Autodesk Inventor part; units mm, degrees
ref_plane "YZ Plane" through (0, 0, 0) normal (1, 0, 0) x (0, 1, 0)
ref_plane "XZ Plane" through (0, 0, 0) normal (0, 1, 0) x (-1, 0, 0)
ref_plane "XY Plane" through (0, 0, 0) normal (0, 0, 1) x (1, 0, 0)
sketch "Sketch1" plane through (0, 0, 0) normal (0, 0, 1) x (1, 0, 0)
  line L0 (-19.05, -19.05) -> (19.05, -19.05)
  line L1 (19.05, -19.05) -> (19.05, 19.05)
  line L2 (19.05, 19.05) -> (-19.05, 19.05)
  line L3 (-19.05, 19.05) -> (-19.05, -19.05)
  line L4 (-19.05, -19.05) -> (19.05, 19.05) construction
  line L5 (19.05, -19.05) -> (-19.05, 19.05) construction
  line L6 (-15.875, -15.875) -> (15.875, -15.875)
  line L7 (15.875, -15.875) -> (15.875, 15.875)
  line L8 (15.875, 15.875) -> (-15.875, 15.875)
  line L9 (-15.875, 15.875) -> (-15.875, -15.875)
  line L10 (-15.875, -15.875) -> (15.875, 15.875) construction
  line L11 (15.875, -15.875) -> (-15.875, 15.875) construction
  point P0 (0, 0)
  dimension "d0" = 38.1
  dimension "d1" = 3.175
extrude "Extrusion1" add sketch "Sketch1" along normal mid plane 304.8
sketch "Sketch3" plane through (0, 0, 152.4) normal (0, 0, 1) x (1, 0, 0)
  line L0 (-19.05, -19.05) -> (19.05, -19.05)
  line L1 (19.05, -19.05) -> (19.05, 19.05)
  line L2 (19.05, 19.05) -> (-19.05, 19.05)
  line L3 (-19.05, 19.05) -> (-19.05, -19.05)
  line L4 (-19.05, -19.05) -> (19.05, 19.05) construction
  line L5 (19.05, -19.05) -> (-19.05, 19.05) construction
  point P0 (0, 0)
extrude "Extrusion2" add sketch "Sketch3" along normal blind 3.175
sketch "Sketch4" plane through (0, 0, 155.575) normal (0, 0, 1) x (1, 0, 0)
  point P0 (0, 0)
  point P1 (0, 0)
hole "Hole1" at (0, 0, 155.575) direction (0, 0, -1) diameter 6.35 end through all
properties part number "LinearExample"
Could you check a few things on this model? Use its own coordinates, in mm. A direction names the side the tool comes from. Give positions to 0.01 mm unless a question says otherwise; leave off trailing zeros. Order: outer loops, then holes, each group sorted by start corner. A loop starts at its lowest first (then second) coordinate and runs counter-clockwise, first axis right, second up.
Item 1: If we mould it in two halves opening along Y, with no side actions, what happens to faces 1 (the face through (-17, 0, -152.4)), 2 (the face through (3.1, 0.69, 153.97)), 3 (the face through (0, -19.05, -1))? For each: pulls with the +Y half, pulls with the -Y half, needs draft (parallel to the pull), parting line crosses it, or undercut.
Item 2: If we section it at C-C, the plane z = -91: Write out the boundary of the cut face in (x, y) (3 decimals).
Item 3: I'm going to push a flat-ended pin straight in: pin 1 (9.5 mm diameter, centred on x = -5.5, y = -7, fed in from -Z). Where does the tip first touch, or does it pass through?
Item 4: If we section it at A-A, the plane x = 0: Write out the boundary of the cut face in (y, z) (3 decimals), plus the area to 3 significant figures.
Item 5: I need wall thicknesses on line 1 (X direction, y = 0, z = 154.1) (3 decimals); line 2 (X direction, y = 9, z = -87) (3 decimals). Which ranges of each line are inside material? Lowest first, please.
Item 6: For faces 4 (the face through (19.05, 0, -1)), 5 (the face through (0, 15.875, -2)), which set-ups out of +Z, -Z, +X, -X, +Y, -Y let a thin tool reach every point of the face, with its end or its side?
Values:
1. face 1: needs draft
1. face 2: undercut
1. face 3: pulls with the -Y half
2. outline: (-19.05, -19.05) - (19.05, -19.05) - (19.05, 19.05) - (-19.05, 19.05) - close; hole (-15.875, -15.875) - (15.875, -15.875) - (15.875, 15.875) - (-15.875, 15.875) - close
3. pin 1: stops at z = 152.4
4. outline: (-19.05, -152.4) - (-15.875, -152.4) - (-15.875, 152.4) - (-3.175, 152.4) - (-3.175, 155.575) - (-19.05, 155.575) - close; (3.175, 152.4) - (15.875, 152.4) - (15.875, -152.4) - (19.05, -152.4) - (19.05, 155.575) - (3.175, 155.575) - close
4. area: 2,040 mm2
5. line 1: x = -19.05 to -3.175, 3.175 to 19.05
5. line 2: x = -19.05 to -15.875, 15.875 to 19.05
6. face 4: +Z, -Z, +X, +Y, -Y
6. face 5: -Z
